Build history of the part. All positions in model axes, mm. A direction names the side the tool comes from. Give positions to 0.01 mm unless a question says otherwise; leave off trailing zeros. Write each loop counter-clockwise with the first axis right and the second up, starting at its lowest first coordinate (ties: lowest second). Pieces come first, ordered by that corner, then holes. Notation, with made-up numbers: (50, 8) -> (54, 8) arc R20 ccw to (54, 15) -> close; hole circle Ø2 at (42.25, 29). An arc over 180 degrees is marked (long way). Put each result on its own line as item: value. Start each with the question number.
Item 1: Slice it at A-A, the plane y = 108. List the corners of the cut face in (x, z).
Item 2: Drill centre lines: line 1 along X through (y, z) = (120.75, 12.7); line 2 along X through (y, z) = (92, 12.5); line 3 along Y through (x, z) = (-44, 7.5). Where is each one in solid material? Low to high.
Item 3: Tool access for faces 1 (the flat face through (5, -21.276, 13)), 2 (the flat face through (3, -24.451, 13)), 3 (the cylindrical face through (92.637, 120.223, 15.132)): list every direction of +Z, -Z, +X, -X, +Y, -Y with a clear straight run to the whole face (end or side of a thin tool).
Item 4: Slice it at D-D, the plane x = -24. List the corners of the cut face in (y, z).
Item 5: Slice it at B-B, the plane z = 12.7. List the corners of the cut face in (x, y), plus the area to 3 significant figures.
Item 6: Flat gauge pins, fed straight in: pin 1 Ø1 at (y, z) = (48.5, 10) entering from -X; pin 2 Ø1.6 at (y, z) = (119.5, 13) entering from -X; pin 3 Ø7.5 at (x, z) = (-78.58, 12.7) entering from +Y. Where does each tip first touch, or does it go through?
Item 7: Two-plate mould, pull along Y, no slides. Class faces 4 (the flat face through (-115.445, 47.689, 12.522)), 5 (the cylindrical face through (-84.92, 120.22, 12.42)), 6 (the flat face through (-119.256, 49.206, 12.522)): pulls with the +Y half, pulls with the -Y half, needs draft (parallel to the pull), parting line crosses it, or undercut.
Item 8: Slice it at C-C, the plane x = -102. List the corners of the cut face in (y, z).
```python
from build123d import *

# Parameters (mm, degrees)
BOSS_EXTRUDE1_DEPTH = 25.4
BOSS_EXTRUDE2_DEPTH = 25.4
SKETCH6_R           = 6.35
CUT_EXTRUDE1_DEPTH  = 10
SKETCH7_R           = 3.675
CUT_EXTRUDE2_DEPTH  = 3.175


with BuildPart() as part:
    # Sketch1 → Boss-Extrude1 (new body)
    with BuildSketch(Plane.XY):
        Polygon((-95.914729745, -24.450906393), (104.110270255, -24.450906393), (150.147770255, 120.829197523), (147.121101424, 121.788312106), (101.785788593, -21.275906393), (-93.590248082, -21.275906393), (-138.925560913, 121.788312106), (-141.952229745, 120.829197523), align=None)
    extrude(amount=BOSS_EXTRUDE1_DEPTH)

    # Sketch4 → Boss-Extrude2 (add)
    with BuildSketch(Plane(origin=(0, 0, 0), x_dir=(-1, 0, 0), z_dir=(0, 0, -1))):
        Polygon((-77.121101424, 121.788312106), (-147.121101424, 121.788312106), (-150.147770255, 120.829197523), (-146.114982495, 118.613312106), (-77.121101424, 118.613312106), align=None)
        Polygon((138.925560913, 121.788312106), (68.925560913, 121.788312106), (68.925560913, 118.613312106), (137.919441985, 118.613312106), (141.952229745, 120.829197523), align=None)
    extrude(amount=-BOSS_EXTRUDE2_DEPTH)

    # Sketch6 → Cut-Extrude1 (cut)
    with BuildSketch(Plane(origin=(0, 121.788312106, 0), x_dir=(1, 0, 0), z_dir=(0, 1, 0))):
        with Locations((-78.575560913, -12.7)):
            Circle(SKETCH6_R)
        with Locations((86.771101424, -12.7)):
            Circle(SKETCH6_R)
    extrude(amount=-CUT_EXTRUDE1_DEPTH, mode=Mode.SUBTRACT)

    # Sketch7 → Cut-Extrude2 (cut)
    with BuildSketch(Plane(origin=(101.650894981, -32.211933717, 0), x_dir=(0, 0, -1), z_dir=(0.953281522, -0.302083333, 0))):
        with Locations((-12.7, 76.285872314)):
            Circle(SKETCH7_R)
    extrude(amount=-CUT_EXTRUDE2_DEPTH, mode=Mode.SUBTRACT)


solid = part.part
```
Values follow:
1. outline: (-137.89, 0) -> (-134.56, 0) -> (-134.56, 25.4) -> (-137.89, 25.4) -> close; (142.75, 0) -> (146.08, 0) -> (146.08, 25.4) -> (142.75, 25.4) -> close
2. line 1: -141.93 to -84.93, -72.23 to -68.93, 77.12 to 80.42, 93.12 to 150.12
2. line 2: -132.82 to -129.49, 137.68 to 141.01
2. line 3: -24.45 to -21.28
3. face 1: +Z, -Z
3. face 2: +Z, -Z, +X, -X, -Y
3. face 3: +Y
4. outline: (-24.45, 0) -> (-21.28, 0) -> (-21.28, 25.4) -> (-24.45, 25.4) -> close
5. outline: (-141.95, 120.83) -> (-95.91, -24.45) -> (104.11, -24.45) -> (123.59, 37.01) -> (120.56, 37.97) -> (101.79, -21.28) -> (-93.59, -21.28) -> (-137.92, 118.61) -> (-84.93, 118.61) -> (-84.93, 121.79) -> (-138.93, 121.79) -> close; (-72.23, 118.61) -> (-68.93, 118.61) -> (-68.93, 121.79) -> (-72.23, 121.79) -> close; (77.12, 118.61) -> (80.42, 118.61) -> (80.42, 121.79) -> (77.12, 121.79) -> close; (93.12, 118.61) -> (146.11, 118.61) -> (122.78, 44.97) -> (125.81, 44.01) -> (150.15, 120.83) -> (147.12, 121.79) -> (93.12, 121.79) -> close
5. area: 1,930 mm2
6. pin 1: x = -119.19
6. pin 2: x = -141.78
6. pin 3: y = -21.28
7. face 4: undercut
7. face 5: needs draft
7. face 6: pulls with the -Y half
8. outline: (-5.25, 0) -> (5.26, 0) -> (5.26, 25.4) -> (-5.25, 25.4) -> close; (118.61, 0) -> (121.79, 0) -> (121.79, 25.4) -> (118.61, 25.4) -> close
